Input: dimensioned drawing with shaded views. Units: mm. Origin: part minimum x, y, z. A direction names the side the tool comes from. Round coordinates to 2 decimals unless told otherwise and drop trailing zeros. Write each loop counter-clockwise with the first axis right and the second up, starting at its lowest first coordinate (ties: lowest second). Pieces come first, ordered by that corner, then holes. Notation, with made-up numbers: (-39, -31) -> (-13, -31) arc R15 cw to (-13, -9) -> close; hole circle Ø6 at (79.25, -28.5). An arc over 180 degrees is marked (long way). Return JSON: item names as keys, results as strings. Group by question number.
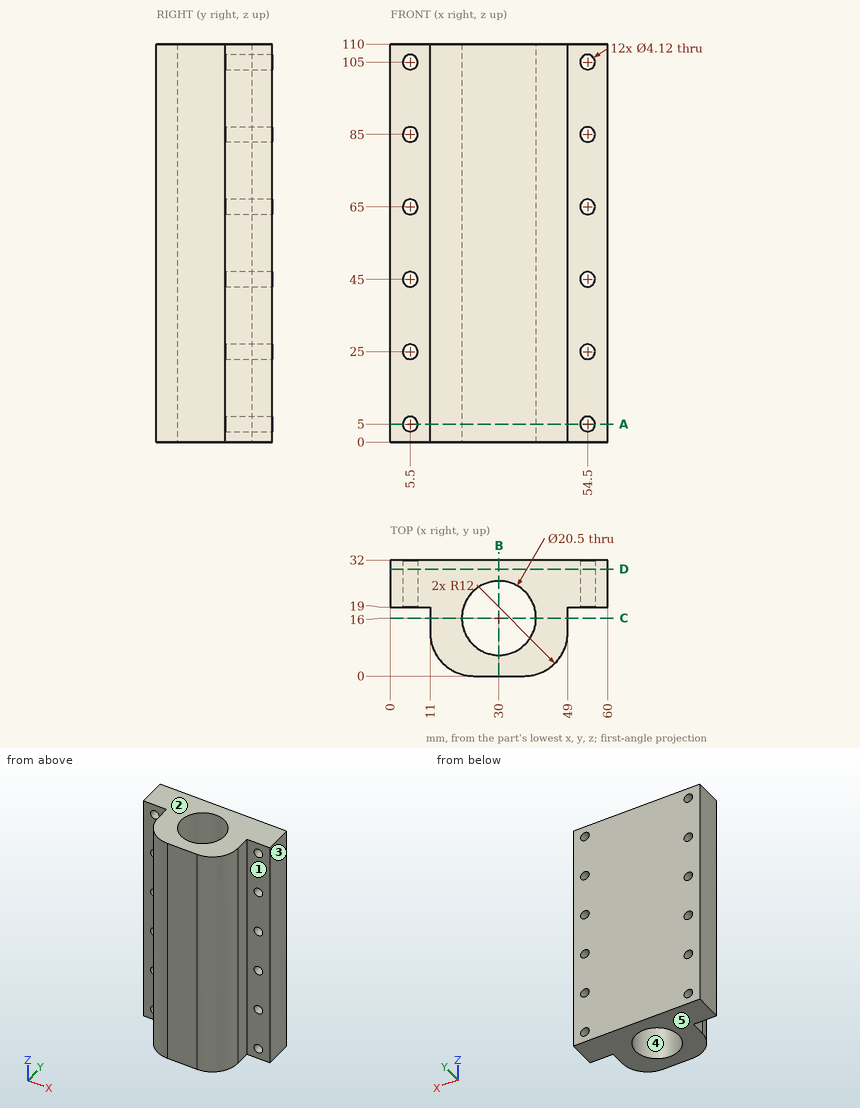
Item 1: Cut plane D-D on y = 29.5. Give the number of separate pieces and of enclosed holes in the cut face, and give its area (3 significant figures).
Item 2: First-contact query: pin 1 Ø5.5 at (x, z) = (54.5, 65) entering from +Y; pin 2 Ø3.5 at (x, z) = (54.5, 25) entering from +Y; pin 3 Ø3.5 at (y, z) = (14.5, 45) entering from +X; pin 4 Ø6.5 at (x, z) = (54.5, 5) entering from -Y. Flat tips, straight axial feed; report the tip coordinate or a pass-through.
Item 3: Cut plane B-B on x = 30. Output: boundary loops of the cut face in (y, z).
Item 4: Pull-direction query (X, two-part tool) for the marked faces 3, 4 and 5; classes: +X half, -X half, draft (parallel to the pull), parting line (faces both ways), or undercut.
Item 5: Material intervals for probe 1 along X at (y, z) = (29, 5); probe 2 along X at (y, z) = (24.5, 65); probe 3 along X at (y, z) = (24, 25), sorted ascending.
Item 6: Cut plane C-C on y = 16. Output: boundary loops of the cut face in (x, z).
Item 7: Set-up query: the marked faces 1 and 2. Return all of +Z, -Z, +X, -X, +Y, -Y with unobstructed straight access to the full face (end or side cutting, diameter ignored); none if empty.
Item 8: Cut plane A-A on z = 5. Output: boundary loops of the cut face in (x, y), and give its area (3 significant figures).
Here are the results:
{
 "1": {"separate pieces": "1", "enclosed holes": "12", "area": "6,440 mm^2"},
 "2": {"pin 1": "stops at y = 32", "pin 2": "passes through", "pin 3": "stops at x = 49", "pin 4": "stops at y = 19"},
 "3": {"outline": "(0, 0) -> (5.75, 0) -> (5.75, 110) -> (0, 110) -> close; (26.25, 0) -> (32, 0) -> (32, 110) -> (26.25, 110) -> close"},
 "4": {"face 3": "+X half", "face 4": "undercut", "face 5": "draft"},
 "5": {"probe 1": "x = 0 to 3.44, 7.56 to 52.44, 56.56 to 60", "probe 2": "x = 0 to 3.44, 7.56 to 24.27, 35.73 to 52.44, 56.56 to 60", "probe 3": "x = 0 to 3.44, 7.56 to 23.59, 36.41 to 52.44, 56.56 to 60"},
 "6": {"outline": "(11, 0) -> (19.75, 0) -> (19.75, 110) -> (11, 110) -> close; (40.25, 0) -> (49, 0) -> (49, 110) -> (40.25, 110) -> close"},
 "7": {"face 1": "+Z, -Z, +X, -Y", "face 2": "+Z, +X, -X, +Y, -Y"},
 "8": {"outline": "(0, 19) -> (3.44, 19) -> (3.44, 32) -> (0, 32) -> close; (7.56, 19) -> (11, 19) -> (11, 12) arc R12 ccw to (23, 0) -> (37, 0) arc R12 ccw to (49, 12) -> (49, 19) -> (52.44, 19) -> (52.44, 32) -> (7.56, 32) -> close; (56.56, 19) -> (60, 19) -> (60, 32) -> (56.56, 32) -> close; hole circle Ø20.5 at (30, 16)", "area": "1,000 mm^2"}
}
